Check sheet for the modelled part. Datum: model origin and axes. Units: mm. A direction names the side the tool comes from. Give positions to 0.01 mm unless a question says otherwise; leave off trailing zeros. Loops run counter-clockwise (first coordinate to the right, second up) from the corner with the lowest first, then second, coordinate; pieces in that order, holes last. Notation, with made-up numbers: (65, -20.75) -> (111, -20.75) arc R28 ccw to (111, 15.25) -> close; hole circle Ø10 at (58.25, 50.5). An arc over 180 degrees is marked (long way). Write each question's results on one line, items separated by ' | '. Start each with the question number.
Item 1: Mould release check, pull along Y, two halves, no side actions. Record for faces 6 (the face through (4, 5.7, 18)), 7 (the face through (-4, 19, -6.7)), 8 (the face through (-6.385, 3.11, 17.249)): pulls with the +Y half, pulls with the -Y half, needs draft (parallel to the pull), parting line crosses it, or undercut.
Item 2: Gauge pin test, flat ends, axial feed: pin 1 Ø4 at (x, z) = (2, 4.5) entering from -Y; pin 2 Ø3 at (x, z) = (2.5, 25.5) entering from +Y; pin 3 Ø12 at (x, y) = (-12, 25) entering from -Z. Record the tip position at first contact, or that the pin passes through.
Item 3: Cross-section at C-C on x = -4. State how many separate pieces and enclosed holes the cut face has, then the cut area to 3 significant figures.
Item 4: Cross-section at A-A on y = 25. Enter the section's corners in (x, z).
Item 5: Access from +Z, -Z, +X, -X, +Y, -Y to the whole of each face (thin tool, end or side, straight path). Record for faces 1 (the face through (-4, 1, 31)), 2 (the face through (-4, 2, -7)), 3 (the face through (-12, 25, -1.3)), 4 (the face through (-4, 5.7, 13)), 5 (the face through (-4, 6, 15)).
Item 6: Cross-section at D-D on z = 22. Enter the section's corners in (x, y).
Item 7: Scan lines: line 1 along X through (y, z) = (3, 18); line 2 along Y through (x, z) = (-4, -4.9); line 3 along Z through (x, y) = (5.5, 15). Record each from-to range of solid material in increasing order.
Item 8: Cross-section at B-B on z = 16. Enter the section's corners in (x, y).
from build123d import *

# Parameters (mm, degrees)
ESBO_O1_W                  = 38
ESBO_O1_H                  = 38
RESSALTO_EXTRUS_O1_DEPTH   = 28
CORTE_EXTRUS_O1_DEPTH      = 57.471231614
ESBO_O7_W                  = 0.3
ESBO_O7_H                  = 28
ESBO_O7_W_2                = 28
ESBO_O7_H_2                = 0.3
ESBO_O7_W_3                = 2
ESBO_O7_H_3                = 2
CORTE_EXTRUS_O2_DEPTH      = 57.471231614
FURO_DE_DI_METRO_7_0_7_3_D = 5
FURO_DE_DI_METRO_7_0_7_2_D = 5
FILETE1_R                  = 4
FILETE2_R                  = 0.15


with BuildPart() as part:
    # Esboço1 → Ressalto-extrusão1 (new body)
    with BuildSketch(Plane(origin=(10, 0, 0), x_dir=(0, 0, -1), z_dir=(1, 0, 0))):
        with Locations((-12, 19)):
            Rectangle(ESBO_O1_W, ESBO_O1_H)
    extrude(amount=-RESSALTO_EXTRUS_O1_DEPTH)

    # Esboço2 → Corte-extrusão1 (cut, through all)
    with BuildSketch(Plane.ZY.offset(18)):
        Polygon((31, 38), (-1, 38), (-1, 12), (5, 6), (31, 6), align=None)
    extrude(amount=-CORTE_EXTRUS_O1_DEPTH, mode=Mode.SUBTRACT)

    # Esboço7 → Corte-extrusão2 (cut, through all)
    with BuildSketch(Plane(origin=(10, 0, 0), x_dir=(0, 0, -1), z_dir=(1, 0, 0))):
        with Locations((6.85, 19)):
            Rectangle(ESBO_O7_W, ESBO_O7_H)
        with Locations((-12, 0.15)):
            Rectangle(ESBO_O7_W_2, ESBO_O7_H_2)
        with Locations((-13, 5.85)):
            Rectangle(ESBO_O7_W_3, ESBO_O7_H_2)
        with Locations((1.15, 20)):
            Rectangle(ESBO_O7_W, ESBO_O7_H_3)
        with Locations((-18, 5.85)):
            Rectangle(ESBO_O7_W_3, ESBO_O7_H_2)
        with Locations((1.15, 25)):
            Rectangle(ESBO_O7_W, ESBO_O7_H_3)
    extrude(amount=-CORTE_EXTRUS_O2_DEPTH, mode=Mode.SUBTRACT)

    # Furo de diâmetro Ø7.0 (7)3 (through all)
    with Locations(Plane(origin=(0, 6, 0), x_dir=(1, 0, 0), z_dir=(0, 1, 0))):
        with Locations((-4, -18)):
            Hole(FURO_DE_DI_METRO_7_0_7_3_D / 2)

    # Furo de diâmetro Ø7.0 (7)2 (through all)
    with Locations(Plane(origin=(0, 0, -7), x_dir=(-1, 0, 0), z_dir=(0, 0, -1))):
        with Locations((4, 25)):
            Hole(FURO_DE_DI_METRO_7_0_7_2_D / 2)

    # Filete1
    filete1_edges = [part.edges().sort_by_distance(p)[0] for p in [
        (-4, 6, 31),
        (-4, 6, 5),
        (-4, 12, -1),
        (-4, 38, -1),
    ]]
    fillet(filete1_edges, radius=FILETE1_R)

    # Filete2
    filete2_edges = [part.edges().sort_by_distance(p)[0] for p in [
        (-4, 5, -7),
        (-4, 5, -6.7),
        (-4, 33, -7),
        (-4, 33, -6.7),
        (-4, 0, 26),
        (-4, 0.3, 26),
        (-4, 0.3, -2),
        (-4, 0, -2),
        (-4, 19, -1.3),
        (-4, 19, -1),
        (-4, 21, -1.3),
        (-4, 21, -1),
        (-4, 5.7, 14),
        (-4, 6, 14),
        (-4, 5.7, 12),
        (-4, 6, 12),
        (-12.145643924, 26, -1.3),
        (-12.145643924, 24, -1.3),
        (-12.145643924, 24, -1),
        (-12.145643924, 26, -1),
        (-12.145643924, 5.7, 19),
        (-12.145643924, 5.7, 17),
        (-12.145643924, 6, 17),
        (-12.145643924, 6, 19),
    ]]
    fillet(filete2_edges, radius=FILETE2_R - 0.0001)  # a hair under: the kernel refuses the full size


solid = part.part
Answer sheet:
1) face 6: pulls with the +Y half | face 7: undercut | face 8: needs draft
2) pin 1: stops at y = 0.3 | pin 2: stops at y = 6 | pin 3: stops at z = -6.7
3) separate pieces: 3 | enclosed holes: 0 | area: 357 mm²
4) outline: (-18, -6.7) -> (-6.5, -6.7) -> (-6.5, -1.3) -> (-18, -1.3) -> close; (-1.5, -6.7) -> (10, -6.7) -> (10, -1.3) -> (-1.5, -1.3) -> close
5) face 1: +Z, +X, -X, +Y, -Y | face 2: -Z, +X, -X, +Y, -Y | face 3: +Z, +X, -X | face 4: +X, -X, +Y | face 5: +Z, +X, -X, +Y
6) outline: (-18, 0.3) -> (10, 0.3) -> (10, 6) -> (-18, 6) -> close
7) line 1: x = -18 to -6.5, -1.5 to 10 | line 2: y = 0 to 22.5, 27.5 to 38 | line 3: z = -6.7 to -1
8) outline: (-18, 0.3) -> (-5.5, 0.3) -> (-5.5, 6) -> (-18, 6) -> close; (-2.5, 0.3) -> (10, 0.3) -> (10, 6) -> (-2.5, 6) -> close
